Work out the finished part from the listing and answer in its coordinate system (mm). A direction names the side the tool comes from. Give positions to 0.01 mm unless a question says otherwise; leave off trailing zeros. Write each loop counter-clockwise with the first axis right and the second up, starting at its lowest first coordinate (ties: lowest second). Pieces come first, ordered by that corner, then holes.
1) Given pin 1 Ø2 at (x, z) = (18.5, -3.5) entering from -Y; pin 2 Ø2 at (x, z) = (30, 0) entering from +Y; pin 3 Ø3 at (y, z) = (1, -0.5) entering from -X; pin 4 Ø5 at (x, z) = (20, -1) entering from +Y, each flat-ended and moving along its own axis, determine where each tip first touches the part or whether it passes through.
2) Straight lines are drawn through the part: probe 1 along Z at (x, y) = (30, 1.85); probe 2 along X at (y, z) = (1.6, 0.75); probe 3 along Z at (x, y) = (0, 2.05). For each, find the intervals that lie inside material, in ascending order.
3) Find section D-D (y = 1.5). Determine the outline of the cut face in (x, z), plus the area to 3 significant figures.
4) Find section C-C (x = 26). Determine the outline of the cut face in (y, z).
5) Find section B-B (z = 0.5). Determine the outline of the cut face in (x, y), plus the area to 3 significant figures.
6) A tool of negligible diameter and unlimited length cuts with its end or side. For faces 4 (the face through (15.019, 4, -3)), 5 (the face through (3.166, 4, 4)), 6 (the face through (14.79, 1.48, 3.76)), from which of +Z, -Z, +X, -X, +Y, -Y can it reach the whole face along a straight path? Write none if from no direction.
7) Find section A-A (y = 4.65). Determine the outline of the cut face in (x, z).
8) Determine the mould class of faces 1 (the face through (24.845, 1.479, 0.479)), 2 (the face through (-1.88, 1.48, 4.09)), 3 (the face through (15.019, 4, 3)) for opening direction X: pulls with the +X half, pulls with the -X half, needs draft (parallel to the pull), parting line crosses it, or undercut.
Autodesk Inventor part; units mm, degrees
ref_plane "YZ Plane" through (0, 0, 0) normal (1, 0, 0) x (0, 1, 0)
ref_plane "XZ Plane" through (0, 0, 0) normal (0, 1, 0) x (-1, 0, 0)
ref_plane "XY Plane" through (0, 0, 0) normal (0, 0, 1) x (1, 0, 0)
sketch "Sketch2" plane through (0, 0, 0) normal (0, 1, 0) x (-1, 0, 0)
  circle A0 centre (0, 0) radius 3.5
  circle A1 centre (0, 0) radius 4.5
  line L0 (0, 0) -> (3.4472, 2.8925)
  line L1 (0, 0) -> (4.5, 0) construction
  line L2 (0, 0) -> (3.4472, -2.8925)
  line L3 (0, 0) -> (4.5, 0) construction
  line L4 (0, 0) -> (-30, 0)
  line L5 (0, 0) -> (30, 0) construction
  circle A2 centre (-30, 0) radius 1.25
  circle A3 centre (-26, 0) radius 1.25
  circle A4 centre (-22, 0) radius 1.25
  circle A5 centre (-30, 0) radius 3
  line L6 (0, 4.5) -> (-30, 3)
  line L7 (-0.0015, -4.5) -> (-30.1494, -2.9963)
  point P0 (2.6812, -2.2498)
  point P1 (2.6812, 2.2498)
  dimension "d11" = 7
  dimension "d12" = 9
  dimension "d13" = 40
  dimension "d14" = 40
  dimension "d15" = 30
  dimension "d16" = 180
  dimension "d17" = 2.5
  dimension "d20" = 4
  dimension "d25" = 6
extrude "Extrusion1" add sketch "Sketch2" along normal blind 3 contours A1 L4 A4 A3 A5 L6 | A0 L4 A1 L0 | L2 A1 L4 A0 | A1 L7 A5 A3 L4 A4 | A5 A3
sketch "Sketch4" plane through (0, 3, 0) normal (0, 1, 0) x (1, 0, 0)
  arc A0 (-2.6812, -2.2498) -> (-2.6812, 2.2498) centre (0, 0) ccw
  line L0 (0, 0) -> (15, 0)
  circle A1 centre (15, 0) radius 2
  circle A2 centre (0, 0) radius 3.5
  line L1 (15.0186, 1.9999) -> (0.3519, 3.4823)
  line L2 (15.0186, -1.9999) -> (0.3519, -3.4823)
  circle A3 centre (15, 0) radius 3.7945
  circle A4 centre (0, 0) radius 4.5
  line L3 (15.0186, 3.7945) -> (0.2127, 4.495)
  line L4 (15.0186, -3.7945) -> (0.2127, -4.495)
  line L5 (3.166, 3.1978) -> (3.166, 4.3552)
  line L6 (3.166, 3.1978) -> (4.3234, 3.1978) construction
  line L7 (3.166, -3.1978) -> (3.166, -4.3552)
  line L8 (3.166, -3.1978) -> (4.3234, -3.1978) construction
  line L9 (15.0186, 1.9999) -> (15.0186, 3.7945)
  line L10 (15.0186, -1.9999) -> (15.0186, -3.7945)
  dimension "d36" = 15
  dimension "d37" = 4
  dimension "d38" = 7
  dimension "d39" = 7.589
  dimension "d40" = 9
  dimension "d41" = 90
  dimension "d42" = 90
extrude "Extrusion2" add sketch "Sketch4" along normal blind 3 contours L2 A3 L4 L7 | L2 L10 A3 | L5 L3 A3 L1 | A3 L9 L1
properties part number "Servo Extension Clip-on"
Results:
1. pin 1: stops at y = 0
1. pin 2: passes through
1. pin 3: stops at x = 2.87
1. pin 4: stops at y = 3
2. probe 1: z = -3 to -1.25, 1.25 to 3
2. probe 2: x = 3.42 to 21, 23 to 25, 27 to 29, 31 to 32.9
2. probe 3: z = -4.5 to -3.5, 3.5 to 4.5
3. outline: (-3.45, -2.89) arc R4.5 ccw to (0, -4.5) - (30.15, -3) arc R3 ccw to (30, 3) - (0, 4.5) arc R4.5 ccw to (-3.45, 2.89) - (-2.68, 2.25) arc R3.5 cw (long way) to (-2.68, -2.25) - close; hole circle Ø2.5 at (22, 0); hole circle Ø2.5 at (26, 0); hole circle Ø2.5 at (30, 0)
3. area: 212 mm2
4. outline: (0, -3.2) - (3, -3.2) - (3, -1.25) - (0, -1.25) - close; (0, 1.25) - (3, 1.25) - (3, 3.2) - (0, 3.2) - close
5. outline: (3.46, 0) - (20.85, 0) - (20.85, 3) - (3.46, 3) - close; (23.15, 0) - (24.85, 0) - (24.85, 3) - (23.15, 3) - close; (27.15, 0) - (28.85, 0) - (28.85, 3) - (27.15, 3) - close; (31.15, 0) - (32.96, 0) - (32.96, 3) - (31.15, 3) - close
5. area: 67.9 mm2
6. face 4: +Z, -Z, +X, +Y
6. face 5: +Z, -Z, -X, +Y
6. face 6: +Z, +X, -Y
7. outline: (3.17, -4.36) - (15.02, -3.79) - (15.02, -2) - (3.17, -3.2) - close; (3.17, 3.2) - (15.02, 2) - (15.02, 3.79) - (3.17, 4.36) - close
8. face 1: undercut
8. face 2: pulls with the -X half
8. face 3: pulls with the +X half
